```python
from build123d import *

# Parameters (mm, degrees)
F0_W      = 34.29
F0_H      = 34.29
F1_DEPTH  = 34.29
F3_R      = 12.7
F4_DEPTH  = 50.8
F5_R      = 3.429
F6_DEPTH  = 25.4
F7_R      = 3.429
F8_DEPTH  = 25.4
F9_R      = 3.429
F10_DEPTH = 25.4
F11_R     = 2.54
F12_R     = 12.7
F13_DEPTH = 50.8
F14_R     = 3.429
F15_DEPTH = 25.4
F16_R     = 2.032
F17_R     = 3.429
F18_DEPTH = 25.4


with BuildPart() as f1:
    # F0 (on Top) → F1 (new body)
    with BuildSketch(Plane.XY):
        with Locations((3.6728888822, 6.5610635031)):
            Rectangle(F0_W, F0_H)
    extrude(amount=F1_DEPTH)

    # F3 (on face) → F4 (join)
    with BuildSketch(Plane.XZ.offset(10.5839364969)):
        with Locations((3.6728888822, 17.145)):
            Circle(F3_R)
    extrude(amount=F4_DEPTH)

    # F5 (on Front) → F6 (cut, symmetric)
    with BuildSketch(Plane.XZ):
        with Locations((3.6728888822, 53.34)):
            Circle(F5_R)
        with Locations((3.6728888822, 72.39)):
            Circle(F5_R)
    extrude(amount=F6_DEPTH, both=True, mode=Mode.SUBTRACT)

    # F7 (on Right) → F8 (cut, symmetric)
    with BuildSketch(Plane.YZ):
        with Locations((-29.6339364969, 17.145)):
            Circle(F7_R)
        with Locations((-48.6839364969, 17.145)):
            Circle(F7_R)
    extrude(amount=F8_DEPTH, both=True, mode=Mode.SUBTRACT)

    # F9 (on Front) → F10 (cut, symmetric)
    with BuildSketch(Plane.XZ):
        with Locations((-51.5721111178, 17.145)):
            Circle(F9_R)
        with Locations((-32.5221111178, 17.145)):
            Circle(F9_R)
    extrude(amount=F10_DEPTH, both=True, mode=Mode.SUBTRACT)

    # F11
    f11_edges = [f1.edges().sort_by_distance(p)[0] for p in [
        (20.817889, 23.706064, 17.145),
        (20.817889, 6.561064, 34.29),
        (20.817889, -10.583936, 17.145),
        (20.817889, 6.561064, 0),
        (3.672889, 23.706064, 0),
        (3.672889, 23.706064, 34.29),
        (-13.472111, 23.706064, 17.145),
        (-13.472111, 6.561064, 0),
        (3.672889, -10.583936, 0),
        (-13.472111, 6.561064, 34.29),
        (-13.472111, -10.583936, 17.145),
        (3.672889, -10.583936, 34.29),
    ]]
    fillet(f11_edges, radius=F11_R)

    # F12 (on face) → F13 (join)
    with BuildSketch(Plane(origin=(0, 23.7060635031, 0), x_dir=(-1, 0, 0), z_dir=(0, 1, 0))):
        with Locations((-3.6728888822, 17.145)):
            Circle(F12_R)
    extrude(amount=F13_DEPTH)

    # F14 (on Right) → F15 (cut, symmetric)
    with BuildSketch(Plane.YZ):
        with Locations((42.7560635031, 17.145)):
            Circle(F14_R)
        with Locations((61.8060635031, 17.145)):
            Circle(F14_R)
    extrude(amount=F15_DEPTH, both=True, mode=Mode.SUBTRACT)

    # F16
    f16_edges = [f1.edges().sort_by_distance(p)[0] for p in [
        (-9.027111, -61.383936, 17.145),
        (16.372889, 74.506064, 17.145),
    ]]
    fillet(f16_edges, radius=F16_R)

    # F17 (on Front) → F18 (cut, symmetric)
    with BuildSketch(Plane.XZ):
        with Locations((58.9178888822, 17.145)):
            Circle(F17_R)
        with Locations((39.8678888822, 17.145)):
            Circle(F17_R)
    extrude(amount=F18_DEPTH, both=True, mode=Mode.SUBTRACT)


solid = f1.part
```
Here's how the part is built. I have some questions about the finished solid (model axes, mm). A direction names the side the tool comes from. Coordinates: 2 decimals unless noted, no trailing zeros. Write each loop counter-clockwise with the first axis right and the second up, starting at its lowest first coordinate (ties: lowest second). Pieces come first, ordered by that corner, then holes. Notation, with made-up numbers: M 24.25,22 L 40.25,22 A13 cw 40.25,44 Z; hole C -23,68 d1. An arc over 180 degrees is marked long. Answer as CSV lines item,"result". Start each with the question number.
Q1. Suppose I cut it at B-B, the plane x = -2. State how many separate pieces and enclosed holes the cut face has, then the cut area to 3 significant figures.
Q2. Suppose I cut it at D-D, the plane y = -29. List the corners of the cut face in (x, z) for me (3 decimals), then the cut area to 3 significant figures.
Q3. Suppose I cut it at A-A, the plane y = -50. List the corners of the cut face in (x, z) for me (3 decimals), then the cut area to 3 significant figures.
Q4. For faces 1 (the cylindrical face through (20.05, 6.77, 33.57)), 2 (the flat face through (3, -10.584, 30)), 3 (the flat face through (3, 23.706, 30)), which set-ups out of +Z, -Z, +X, -X, +Y, -Y let a thin tool reach every point of the face, with its end or its side?
Q5. If we mould it in two halves opening along Y, with no side actions, what happens to faces 4 (the cylindrical face through (20.054, -9.86, 17.349)), 5 (the cylindrical face through (3.85, 65.08, 18.17)), 6 (the cylindrical face through (20.05, 6.77, 0.72))? For each: pulls with the +Y half, pulls with the -Y half, needs draft (parallel to the pull), parting line crosses it, or undercut.
Q6. Will these pins go through, and if not, where does the flat tip stop? pin 1 Ø8 at (y, z) = (-29.63, 17.14) entering from +X; pin 2 Ø6 at (y, z) = (42.76, 17.14) entering from -X; pin 3 Ø4 at (x, y) = (-3, -47) entering from +Z; pin 4 Ø12 at (y, z) = (-34, 24) entering from -X.
Q7. I need wall thicknesses on probe 1 along Y at (x, z) = (-1, 18); probe 2 along X at (y, z) = (48, 18); probe 3 along Z at (x, y) = (4.5, 29.5). Which ranges of each line are inside material? Lowest first, please. Write a range as [from, to].
Entries:
1,separate pieces,"1"
1,enclosed holes,"4"
1,area,"3,330 mm²"
2,outline,"M -8.572,13.775 A12.7 ccw 15.918,13.775 Z; M -8.572,20.515 L 15.918,20.515 A12.7 ccw Z"
2,area,"338 mm²"
3,outline,"M -8.626,13.979 A12.7 ccw 15.972,13.979 Z; M -8.626,20.311 L 15.972,20.311 A12.7 ccw Z"
3,area,"348 mm²"
4,face 1,"+Z, +X, +Y, -Y"
4,face 2,"-Y"
4,face 3,"+Y"
5,face 4,"pulls with the -Y half"
5,face 5,"undercut"
5,face 6,"needs draft"
6,pin 1,"stops at x = 16.37"
6,pin 2,"passes through"
6,pin 3,"stops at z = 28.95"
6,pin 4,"stops at x = -9"
7,probe 1,"y = [-61.38, -52], [-45.36, -32.95], [-26.31, 39.44], [46.08, 58.49], [65.13, 74.51]"
7,probe 2,"x = [-9, 16.34]"
7,probe 3,"z = [4.47, 29.82]"
